from build123d import *

# Parameters (mm, degrees)
SKETCH1_R           = 50.1
BOSS_EXTRUDE5_DEPTH = 25.3
SKETCH4_R           = 30.6
CUT_EXTRUDE1_DEPTH  = 7.6
CUT_EXTRUDE2_START  = -7.6
SKETCH5_R           = 30.6
CUT_EXTRUDE2_DEPTH  = 7.6
SKETCH6_R           = 10
BOSS_EXTRUDE7_DEPTH = 7.6
SKETCH7_R           = 5.05
CUT_EXTRUDE5_DEPTH  = 10000
BOSS_EXTRUDE8_START = 2
BOSS_EXTRUDE8_DEPTH = 2
SKETCH9_R           = 2.5
CUT_EXTRUDE11_DEPTH = 74.029514581


with BuildPart() as part:
    # Sketch1 → Boss-Extrude5 (new body)
    with BuildSketch(Plane.XY):
        Circle(SKETCH1_R)
    extrude(amount=BOSS_EXTRUDE5_DEPTH)

    # Sketch4 → Cut-Extrude1 (cut)
    with BuildSketch(Plane.XY.offset(25.3)):
        Circle(SKETCH4_R)
    extrude(amount=-CUT_EXTRUDE1_DEPTH, mode=Mode.SUBTRACT)

    # Sketch5 → Cut-Extrude2 (cut)
    with BuildSketch(Plane(origin=(0, 0, 0), x_dir=(-1, 0, 0), z_dir=(0, 0, -1)).offset(CUT_EXTRUDE2_START)):
        with Locations(Location((0, 0, 0), (0, 0, 180))):
            Circle(SKETCH5_R)
    extrude(amount=CUT_EXTRUDE2_DEPTH, mode=Mode.SUBTRACT)

    # Sketch6 → Boss-Extrude7 (add)
    with BuildSketch(Plane.XY.offset(17.7)):
        with Locations(Location((0, 0, 0), (0, 0, 180))):
            Circle(SKETCH6_R)
    extrude(amount=BOSS_EXTRUDE7_DEPTH)

    # Sketch7 → Cut-Extrude5 (cut)
    with BuildSketch(Plane.XY.offset(25.3)):
        Circle(SKETCH7_R)
    extrude(amount=-CUT_EXTRUDE5_DEPTH, mode=Mode.SUBTRACT)

    # Sketch8 → Boss-Extrude8 (add)
    with BuildSketch(Plane.XY.offset(17.7).offset(BOSS_EXTRUDE8_START)):
        with BuildLine():
            Line((-30.6, 0), (-10, 0))
            ThreePointArc((-10, 0), (-9.985723513, -0.534159082), (-9.942934815, -1.066792981))
            Line((-9.942934815, -1.066792981), (-30.581398803, -1.066792981))
            ThreePointArc((-30.581398803, -1.066792981), (-30.595349347, -0.53347757), (-30.6, 0))
        make_face()
        with BuildLine():
            Line((-16.214569224, 25.950871756), (-5.89533723, 8.077437647))
            ThreePointArc((-5.89533723, 8.077437647), (-5.455457091, 8.380810696), (-5, 8.660254038))
            Line((-5, 8.660254038), (-15.3, 26.500377356))
            ThreePointArc((-15.3, 26.500377356), (-15.759679801, 26.229610988), (-16.214569224, 25.950871756))
        make_face()
        with BuildLine():
            Line((14.366829579, 27.017664737), (4.047597585, 9.144230629))
            ThreePointArc((4.047597585, 9.144230629), (4.530266422, 8.914969778), (5, 8.660254038))
            Line((5, 8.660254038), (15.3, 26.500377356))
            ThreePointArc((15.3, 26.500377356), (14.835669546, 26.763088557), (14.366829579, 27.017664737))
        make_face()
        with BuildLine():
            Line((30.581398803, 1.066792981), (9.942934815, 1.066792981))
            ThreePointArc((9.942934815, 1.066792981), (9.985723513, 0.534159082), (10, 0))
            Line((10, 0), (30.6, 0))
            ThreePointArc((30.6, 0), (30.595349347, 0.53347757), (30.581398803, 1.066792981))
        make_face()
        with BuildLine():
            Line((16.214569224, -25.950871756), (5.89533723, -8.077437647))
            ThreePointArc((5.89533723, -8.077437647), (5.455457091, -8.380810696), (5, -8.660254038))
            Line((5, -8.660254038), (15.3, -26.500377356))
            ThreePointArc((15.3, -26.500377356), (15.759679801, -26.229610988), (16.214569224, -25.950871756))
        make_face()
        with BuildLine():
            Line((-14.366829579, -27.017664737), (-4.047597585, -9.144230629))
            ThreePointArc((-4.047597585, -9.144230629), (-4.530266422, -8.914969778), (-5, -8.660254038))
            Line((-5, -8.660254038), (-15.3, -26.500377356))
            ThreePointArc((-15.3, -26.500377356), (-14.835669546, -26.763088557), (-14.366829579, -27.017664737))
        make_face()
    extrude(amount=-BOSS_EXTRUDE8_DEPTH)

    # Sketch9 → Cut-Extrude11 (cut, through all)
    with BuildSketch(Plane.XY.offset(7.6)):
        with Locations((-19.982206185, -12.462368817)):
            Circle(SKETCH9_R)
        with Locations((-20.783831079, 11.073913771)):
            Circle(SKETCH9_R)
        with Locations((-0.801624894, 23.536282588)):
            Circle(SKETCH9_R)
        with Locations((19.982206185, 12.462368817)):
            Circle(SKETCH9_R)
        with Locations((20.783831079, -11.073913771)):
            Circle(SKETCH9_R)
        with Locations((0.801624894, -23.536282588)):
            Circle(SKETCH9_R)
    extrude(amount=CUT_EXTRUDE11_DEPTH, mode=Mode.SUBTRACT)


solid = part.part
The model under review builds one solid part; all positions refer to its coordinate system, in mm. A direction names the side the tool comes from. Give positions to 0.01 mm unless a question says otherwise; leave off trailing zeros. Order: outer loops, then holes, each group sorted by start corner. A loop starts at its lowest first (then second) coordinate and runs counter-clockwise, first axis right, second up. Notation, with made-up numbers: M 84.5,5.5 L 137.5,5.5 A15 cw 137.5,29.5 Z; hole C 80,52 d11. An arc over 180 degrees is marked long. Use one line per item in the form item = value. Start each with the question number.
Item 1: For faces 3 (the cylindrical face through (0.26, -25.977, 12.579)), 4 (the flat face through (-11.127, 17.139, 18.714)), 5 (the flat face through (6, 0, 7.6)), list the 3-axis set-ups (+Z, -Z, +X, -X, +Y, -Y) from which the entire face can be reached by the end or side of a thin tool; tool diameter is ignored.
Item 2: Insertion check: pin 1 Ø6 at (y, z) = (24.5, 12) entering from +X; pin 2 Ø1 at (y, z) = (-21.5, 9.5) entering from +X; pin 3 Ø9 at (x, y) = (11, -20) entering from +Z; pin 4 Ø6 at (x, y) = (0, 0) entering from +Z. Each pin has a flat end and moves straight along its axis. Give the tip position at first contact, or say it passes through.
Item 3: We need section C-C on y = -2.5. Give the boundary of the cut face in (x, z).
Item 4: To check wall thickness, follow line 1 along Y through (x, z) = (8, 21); line 2 along Y through (x, z) = (2, 11.75); line 3 along X through (y, z) = (11.5, 20). State the ranges of each line that lie inside material, in increasing order. Write a range as from..to.
Item 5: We need section A-A on z = 12. Give the boundary of the cut face in (x, y).
Item 6: We need section B-B on x = 0. Give the boundary of the cut face in (y, z), plus the area to 3 significant figures.
Item 7: The part is to be moulded in two halves that separate along X. For faces 1 (the flat face through (2, -5, 25.3)), 2 (the flat face through (10.08, 17.46, 18.71)), say which applies: pulls with the +X half, pulls with the -X half, needs draft (parallel to the pull), parting line crosses it, or undercut.
Item 8: We need section D-D on z = 23.75. Give the boundary of the cut face in (x, y).
Completed:
q1.face_3 = +Z, -Z
q1.face_4 = +Z
q1.face_5 = -Z
q2.pin_1 = 45.25
q2.pin_2 = 45.49
q2.pin_3 = 19.7
q2.pin_4 = through
q3.outline = M -50.04,0 L -30.5,0 L -30.5,7.6 L -4.39,7.6 L -4.39,25.3 L -9.68,25.3 L -9.68,17.7 L -30.5,17.7 L -30.5,25.3 L -50.04,25.3 Z; M 4.39,7.6 L 30.5,7.6 L 30.5,0 L 50.04,0 L 50.04,25.3 L 30.5,25.3 L 30.5,17.7 L 9.68,17.7 L 9.68,25.3 L 4.39,25.3 Z
q4.line_1 = -49.46..-29.54, -6..6, 29.54..49.46
q4.line_2 = -50.06..-25.73, -21.34..-4.64, 4.64..50.06
q4.line_3 = -48.76..-28.36, 28.36..48.76
q5.outline = C 0,0 d100.2; hole C -20.78,11.07 d5; hole C -19.98,-12.46 d5; hole C 0,0 d10.1; hole C -0.8,23.54 d5; hole C 0.8,-23.54 d5; hole C 19.98,12.46 d5; hole C 20.78,-11.07 d5
q6.outline = M -50.1,0 L -30.6,0 L -30.6,7.6 L -25.9,7.6 L -25.9,17.7 L -30.6,17.7 L -30.6,25.3 L -50.1,25.3 Z; M -21.17,7.6 L -5.05,7.6 L -5.05,25.3 L -10,25.3 L -10,17.7 L -21.17,17.7 Z; M 5.05,7.6 L 21.17,7.6 L 21.17,17.7 L 10,17.7 L 10,25.3 L 5.05,25.3 Z; M 25.9,7.6 L 30.6,7.6 L 30.6,0 L 50.1,0 L 50.1,25.3 L 30.6,25.3 L 30.6,17.7 L 25.9,17.7 Z
q6.area = 1,480 mm²
q7.face_1 = needs draft
q7.face_2 = undercut
q8.outline = C 0,0 d100.2; C 0,0 d20; hole C 0,0 d61.2; hole C 0,0 d10.1
